from build123d import *

# Parameters (mm, degrees)
SKETCH1_W           = 16.9
SKETCH1_H           = 20.5
BOSS_EXTRUDE1_DEPTH = 1.5
SKETCH2_W           = 16.9
SKETCH2_H           = 20.5
BOSS_EXTRUDE2_DEPTH = 8.6
FILLET1_R           = 3
FILLET2_R           = 1
SKETCH3_R           = 1.5
CUT_EXTRUDE1_DEPTH  = 10


with BuildPart() as part:
    # Sketch1 → Boss-Extrude1 (new body)
    with BuildSketch(Plane(origin=(0, 0, 0), x_dir=(1, 0, 0), z_dir=(0, 1, 0))):
        with BuildLine():
            Line((-8.45, 3.25), (-8.45, 8.25))
            Line((-8.45, 8.25), (-12.45, 8.25))
            Line((-12.45, 8.25), (-12.45, 6.9))
            Line((-12.45, 6.9), (-9.75, 6.9))
            ThreePointArc((-9.75, 6.9), (-8.936827202, 6.563172798), (-8.6, 5.75))
            ThreePointArc((-8.6, 5.75), (-8.936827202, 4.936827202), (-9.75, 4.6))
            Line((-9.75, 4.6), (-12.45, 4.6))
            Line((-12.45, 4.6), (-12.45, 3.25))
            Line((-12.45, 3.25), (-8.45, 3.25))
        make_face()
        Rectangle(SKETCH1_W, SKETCH1_H)
        with BuildLine():
            Line((12.45, 8.25), (8.45, 8.25))
            Line((8.45, 8.25), (8.45, 3.25))
            Line((8.45, 3.25), (12.45, 3.25))
            Line((12.45, 3.25), (12.45, 4.6))
            Line((12.45, 4.6), (9.75, 4.6))
            ThreePointArc((9.75, 4.6), (8.6, 5.75), (9.75, 6.9))
            Line((9.75, 6.9), (12.45, 6.9))
            Line((12.45, 6.9), (12.45, 8.25))
        make_face()
    extrude(amount=BOSS_EXTRUDE1_DEPTH)

    # Sketch2 → Boss-Extrude2 (add)
    with BuildSketch(Plane(origin=(0, 1.5, 0), x_dir=(1, 0, 0), z_dir=(0, 1, 0))):
        Rectangle(SKETCH2_W, SKETCH2_H)
    extrude(amount=BOSS_EXTRUDE2_DEPTH)

    # Fillet1
    fillet1_edges = [part.edges().sort_by_distance(p)[0] for p in [
        (8.45, 5.05, 10.25),
        (-8.45, 5.05, 10.25),
        (-8.45, 10.1, 0),
        (0, 10.1, 10.25),
        (8.45, 10.1, 0),
    ]]
    fillet(fillet1_edges, radius=FILLET1_R)

    # Fillet2
    fillet2_edges = [part.edges().sort_by_distance(p)[0] for p in [
        (-12.45, 0.75, -8.25),
        (-8.45, 0.75, -8.25),
        (8.45, 0.75, -8.25),
        (12.45, 0.75, -8.25),
        (12.45, 0.75, -3.25),
        (8.45, 0.75, -3.25),
        (-8.45, 0.75, -3.25),
        (-12.45, 0.75, -3.25),
    ]]
    fillet(fillet2_edges, radius=FILLET2_R)

    # Sketch3 → Cut-Extrude1 (cut)
    with BuildSketch(Plane(origin=(0, 0, -10.25), x_dir=(-1, 0, 0), z_dir=(0, 0, -1))):
        Polygon((7.5, 4.05), (7.5, 6.05), (6, 7.55), (-7.5, 7.55), (-7.5, 2.55), (6, 2.55), align=None)
        with Locations((-3.6, 5.05)):
            Circle(SKETCH3_R, mode=Mode.SUBTRACT)
        with Locations((3.6, 5.05)):
            Circle(SKETCH3_R, mode=Mode.SUBTRACT)
    extrude(amount=-CUT_EXTRUDE1_DEPTH, mode=Mode.SUBTRACT)


solid = part.part
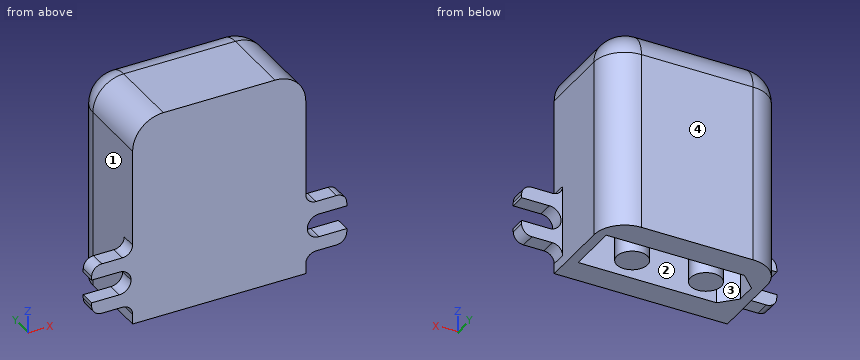
Verification items for the finished model (mm, model axes). Face numbers are marked on the shaded views. Give positions to 0.01 mm unless a question says otherwise; leave off trailing zeros. Write each loop counter-clockwise with the first axis right and the second up, starting at its lowest first coordinate (ties: lowest second). Pieces come first, ordered by that corner, then holes.
(1) Cross-section at C-C (z = -2.75). Enter the section's corners in (x, y), plus the area to 3 significant figures.
(2) Gauge pin test, flat ends, axial feed: pin 1 (2 mm diameter, centred on x = 7.5, y = 1.5, fed in from +Z); pin 2 (3 mm diameter, centred on y = 2.5, z = 5.5, fed in from -X); pin 3 (0.8 mm diameter, centred on x = -10, y = 1, fed in from -Z). Record the tip position at first contact, or that the pin passes through.
(3) Mould release check, pull along X, two halves, no side actions. Record for the marked faces 1, 2, 3 and 4: +X half, -X half, draft (parallel to the pull), parting line (faces both ways), or undercut.
(4) Cross-section at A-A (x = 10.25). Enter the section's corners in (y, z).
(5) Material ranges on line 1 (Y direction, x = 1.25, z = -7); line 2 (Y direction, x = -3, z = -2.25); line 3 (Y direction, x = -3.25, z = -1), recorded low to high.
(6) Cross-section at D-D (x = 3.6). Enter the section's corners in (y, z).
(7) Cross-section at B-B (y = 5.05). Enter the section's corners in (x, z), plus the area to 3 significant figures.
Worked out:
1. outline: (-8.58, 0) - (8.58, 0) - (8.58, 1.5) - (8.45, 1.5) - (8.45, 7.1) arc R3 ccw to (5.45, 10.1) - (-5.45, 10.1) arc R3 ccw to (-8.45, 7.1) - (-8.45, 1.5) - (-8.58, 1.5) - close; circle Ø3 at (-3.6, 5.05); circle Ø3 at (3.6, 5.05); hole (-7.5, 4.05) - (-6, 2.55) - (7.5, 2.55) - (7.5, 7.55) - (-6, 7.55) - (-7.5, 6.05) - close
1. area: 109 mm2
2. pin 1: stops at z = 10.06
2. pin 2: stops at x = -8.45
2. pin 3: stops at z = -8.25
3. face 1: -X half
3. face 2: undercut
3. face 3: undercut
3. face 4: draft
4. outline: (0, -8.25) - (1.5, -8.25) - (1.5, -6.9) - (0, -6.9) - close; (0, -4.6) - (1.5, -4.6) - (1.5, -3.25) - (0, -3.25) - close
5. line 1: y = 0 to 2.55, 7.55 to 10.1
5. line 2: y = 0 to 2.55, 3.68 to 6.42, 7.55 to 10.1
5. line 3: y = 0 to 2.55, 3.59 to 6.51, 7.55 to 10.1
6. outline: (0, -10.25) - (2.55, -10.25) - (2.55, -0.25) - (3.55, -0.25) - (3.55, -10.25) - (6.55, -10.25) - (6.55, -0.25) - (7.55, -0.25) - (7.55, -10.25) - (10.1, -10.25) - (10.1, 7.25) arc R3 ccw to (7.1, 10.25) - (0, 10.25) - close
7. outline: (-8.45, -10.25) - (-7.5, -10.25) - (-7.5, -0.25) - (-5.1, -0.25) - (-5.1, -10.25) - (-2.1, -10.25) - (-2.1, -0.25) - (2.1, -0.25) - (2.1, -10.25) - (5.1, -10.25) - (5.1, -0.25) - (7.5, -0.25) - (7.5, -10.25) - (8.45, -10.25) - (8.45, 7.25) arc R3 ccw to (5.45, 10.25) - (-5.45, 10.25) arc R3 ccw to (-8.45, 7.25) - close
7. area: 253 mm2
